```python
from build123d import *

# Parameters (mm, degrees)
F1_DEPTH = 6
F2_DEPTH = 4
F3_DEPTH = 2


with BuildPart() as f1:
    # F0 (on Top) → F1 (new body)
    with BuildSketch(Plane.XY):
        with BuildLine():
            Line((0, -75), (71.3659359191, 15.1770657673))
            ThreePointArc((71.3659359191, 15.1770657673), (53.1408249977, 77.7798718682), (0, 40))
            ThreePointArc((0, 40), (-53.1408249977, 77.7798718682), (-71.3659359191, 15.1770657673))
            Line((-71.3659359191, 15.1770657673), (0, -75))
        make_face()
        with BuildLine():
            ThreePointArc((-62.3608017817, 13.1737193764), (-46.5622648655, 68.0350424728), (0, 35))
            ThreePointArc((0, 35), (46.5622648655, 68.0350424728), (62.3608017817, 13.1737193764))
            Line((62.3608017817, 13.1737193764), (35, -21.125))
            Line((35, -21.125), (23.9316239316, -35))
            Line((23.9316239316, -35), (0, -65))
            Line((0, -65), (-62.3608017817, 13.1737193764))
        make_face(mode=Mode.SUBTRACT)
    extrude(amount=-F1_DEPTH)

    # F0 (on Top) → F2 (join)
    with BuildSketch(Plane.XY):
        with BuildLine():
            ThreePointArc((62.3608017817, 13.1737193764), (46.5622648655, 68.0350424728), (0, 35))
            ThreePointArc((0, 35), (-46.5622648655, 68.0350424728), (-62.3608017817, 13.1737193764))
            Line((-62.3608017817, 13.1737193764), (0, -65))
            Line((0, -65), (23.9316239316, -35))
            Line((23.9316239316, -35), (35, -21.125))
            Line((35, -21.125), (62.3608017817, 13.1737193764))
        make_face()
        with BuildLine():
            Line((35, 6.6666666667), (0, -40))
            Line((0, -40), (-36, 8))
            ThreePointArc((-36, 8), (-26.3245553203, 38.973665961), (0, 20))
            ThreePointArc((0, 20), (26.3245553203, 38.973665961), (36, 8))
            Line((36, 8), (35, 6.6666666667))
        make_face(mode=Mode.SUBTRACT)
    extrude(amount=-F2_DEPTH)

    # F0 (on Top) → F3 (join)
    with BuildSketch(Plane.XY):
        with BuildLine():
            Line((-36, 8), (0, -40))
            Line((0, -40), (35, 6.6666666667))
            Line((35, 6.6666666667), (35, 6.7712434447))
            ThreePointArc((35, 6.7712434447), (35.5121713718, 7.3757162844), (36, 8))
            ThreePointArc((36, 8), (26.3245553203, 38.973665961), (0, 20))
            ThreePointArc((0, 20), (-26.3245553203, 38.973665961), (-36, 8))
        make_face()
    extrude(amount=-F3_DEPTH)


solid = f1.part
```
Build history of the part. All positions in model axes, mm. A direction names the side the tool comes from. Round coordinates to 2 decimals unless told otherwise and drop trailing zeros. Write each loop counter-clockwise with the first axis right and the second up, starting at its lowest first coordinate (ties: lowest second). Pieces come first, ordered by that corner, then holes.
1) Band-saw the part on B-B, the plane x = -20.5. List the corners of the cut face in (y, z), and give its area (3 significant figures).
2) Pin check, flat tips, straight feed: pin 1 (1 mm diameter, centred on x = -38.5, z = -4.5, fed in from -Y); pin 2 (6 mm diameter, centred on x = 10, y = -44, fed in from -Z); pin 3 (3 mm diameter, centred on y = -26, z = -3, fed in from +X). Stop position of each tip, or through.
3) Mould opens along X. For faces 1 (the flat face through (-1, 21, 0)), 2 (the flat face through (35.183, -30.543, -2.958)), 3 (the cylindrical face through (-47.44, 67.715, -4.986)), 4 (the flat face through (-36.183, -29.28, -2.958)) say: +X half, -X half, draft (parallel to the pull), parting line (faces both ways), or undercut.
4) Band-saw the part on C-C, the plane y = -37. List the corners of the cut face in (x, z).
5) Band-saw the part on A-A, the plane z = -4.9. List the corners of the cut face in (x, y) (3 decimals).
6) Drill centre lines: probe 1 along X at (y, z) = (61, -5.5); probe 2 along Z at (x, y) = (16, 40); probe 3 along Y at (x, z) = (20, -2.8). Where is each one in solid material? Low to high.
7) 3-axis set-ups, long thin cutter, end or side, ignore diameter. For faces 5 (the flat face through (-1, 9, -2)), 6 (the flat face through (-0.4, 43, -6)): which of +Z, -Z, +X, -X, +Y, -Y reach the whole face in a straight line?
Ans:
1. outline: (-49.1, -6) - (-39.3, -6) - (-39.3, -4) - (-12.67, -4) - (-12.67, -2) - (39.99, -2) - (39.99, -4) - (66.86, -4) - (66.86, -6) - (74.92, -6) - (74.92, 0) - (-49.1, 0) - close
1. area: 426 mm2
2. pin 1: stops at y = -26.98
2. pin 2: stops at z = -4
2. pin 3: stops at x = 39.97
3. face 1: draft
3. face 2: +X half
3. face 3: undercut
3. face 4: -X half
4. outline: (-30.07, -6) - (-22.34, -6) - (-22.34, -4) - (-2.25, -4) - (-2.25, -2) - (2.25, -2) - (2.25, -4) - (22.34, -4) - (22.34, -6) - (30.07, -6) - (30.07, 0) - (-30.07, 0) - close
5. outline: (-71.366, 15.177) - (0, -75) - (71.366, 15.177) arc R40 ccw (long way) to (0, 40) arc R40 ccw (long way) to start; hole (-62.361, 13.174) - (0, -65) - (62.361, 13.174) arc R35 ccw (long way) to (0, 35) arc R35 ccw (long way) to start
6. probe 1: x = -74.04 to -58.43, -11.57 to -5.96, 5.96 to 11.57, 58.43 to 74.04
6. probe 2: z = -4 to 0
6. probe 3: y = -49.73 to -13.33, 40 to 74.64
7. face 5: -Z
7. face 6: -Z, +X, -X, +Y, -Y
